Can you work these out from the model? Positions are in its coordinate system, mm. A direction names the side the tool comes from. Give positions to 0.01 mm unless a question says otherwise; leave off trailing zeros. Answer as a JSON object with one key per item and string values.
Autodesk Inventor part; units mm, degrees
ref_plane "YZ Plane" through (0, 0, 0) normal (1, 0, 0) x (0, 1, 0)
ref_plane "XZ Plane" through (0, 0, 0) normal (0, 1, 0) x (-1, 0, 0)
ref_plane "XY Plane" through (0, 0, 0) normal (0, 0, 1) x (1, 0, 0)
sketch "Szkic1" plane through (0, 0, 0) normal (0, 1, 0) x (-1, 0, 0)
  line L0 (35.259, 49.5664) -> (-29.741, 49.5664)
  line L1 (-29.741, 49.5664) -> (-29.741, 19.5664)
  line L2 (-29.741, 19.5664) -> (35.259, 19.5664)
  line L3 (35.259, 19.5664) -> (35.259, 49.5664)
  point P0 (0, 0)
  dimension "d0" = 65
  dimension "d1" = 30
extrude "Wyciągnięcie proste1" add sketch "Szkic1" along normal blind 1.6
fillet "Zaokrąglenie1" radius 2 4 edges at (-35.259, 0.8, 19.5664) (-35.259, 0.8, 49.5664) (29.741, 0.8, 49.5664) (29.741, 0.8, 19.5664)
sketch "Szkic2" plane through (0, 1.6, 0) normal (0, 1, 0) x (1, 0, 0)
  arc A0 (29.741, -21.5664) -> (27.741, -19.5664) centre (27.741, -21.5664) ccw
  line L0 (27.741, -19.5664) -> (-33.259, -19.5664)
  arc A1 (-33.259, -19.5664) -> (-35.259, -21.5664) centre (-33.259, -21.5664) ccw
  line L1 (-35.259, -21.5664) -> (-35.259, -47.5664)
  arc A2 (-35.259, -47.5664) -> (-33.259, -49.5664) centre (-33.259, -47.5664) ccw
  line L2 (-33.259, -49.5664) -> (27.741, -49.5664)
  arc A3 (27.741, -49.5664) -> (29.741, -47.5664) centre (27.741, -47.5664) ccw
  line L3 (29.741, -47.5664) -> (29.741, -21.5664)
  line L4 (-33.259, -20.0664) -> (27.741, -20.0664)
  arc A4 (29.241, -21.5664) -> (27.741, -20.0664) centre (27.741, -21.5664) ccw
  line L5 (29.241, -21.5664) -> (29.241, -47.5664)
  arc A5 (27.741, -49.0664) -> (29.241, -47.5664) centre (27.741, -47.5664) ccw
  line L6 (27.741, -49.0664) -> (-33.259, -49.0664)
  arc A6 (-34.759, -47.5664) -> (-33.259, -49.0664) centre (-33.259, -47.5664) ccw
  line L7 (-34.759, -47.5664) -> (-34.759, -21.5664)
  arc A7 (-33.259, -20.0664) -> (-34.759, -21.5664) centre (-33.259, -21.5664) ccw
  point P0 (0, 0)
  dimension "d5" = 0.5
extrude "Wyciągnięcie proste2" cut sketch "Szkic2" against normal through all
sketch "Szkic3" plane through (0, 1.6, 0) normal (0, 1, 0) x (1, 0, 0)
  line L0 (-19.799, -32.0164) -> (-20.439, -32.0164)
  line L1 (-20.439, -32.0164) -> (-20.439, -31.3764)
  line L2 (-19.799, -31.3764) -> (-19.799, -32.0164)
  line L3 (-20.439, -31.3764) -> (-19.799, -31.3764)
  line L4 (-19.799, -29.4764) -> (-20.439, -29.4764)
  line L5 (-19.799, -28.8364) -> (-19.799, -29.4764)
  line L6 (-20.439, -29.4764) -> (-20.439, -28.8364)
  line L7 (-20.439, -28.8364) -> (-19.799, -28.8364)
  line L8 (-19.799, -26.9364) -> (-20.439, -26.9364)
  line L9 (-19.799, -26.2964) -> (-19.799, -26.9364)
  line L10 (-20.439, -26.9364) -> (-20.439, -26.2964)
  line L11 (-20.439, -26.2964) -> (-19.799, -26.2964)
  line L12 (-20.439, -24.3964) -> (-20.439, -23.7564)
  line L13 (-19.799, -24.3964) -> (-20.439, -24.3964)
  line L14 (-20.439, -23.7564) -> (-19.799, -23.7564)
  line L15 (-19.799, -23.7564) -> (-19.799, -24.3964)
  line L16 (-17.469, -25.4431) -> (-16.829, -25.4431)
  line L17 (-17.469, -26.0831) -> (-17.469, -25.4431)
  line L18 (-16.829, -26.0831) -> (-17.469, -26.0831)
  line L19 (-16.829, -25.4431) -> (-16.829, -26.0831)
  line L20 (-14.929, -26.0831) -> (-14.929, -25.4431)
  line L21 (-14.289, -26.0831) -> (-14.929, -26.0831)
  line L22 (-14.929, -25.4431) -> (-14.289, -25.4431)
  line L23 (-14.289, -25.4431) -> (-14.289, -26.0831)
  line L24 (-12.389, -26.0831) -> (-12.389, -25.4431)
  line L25 (-11.749, -26.0831) -> (-12.389, -26.0831)
  line L26 (-12.389, -25.4431) -> (-11.749, -25.4431)
  line L27 (-11.749, -25.4431) -> (-11.749, -26.0831)
  line L28 (-9.849, -26.0831) -> (-9.849, -25.4431)
  line L29 (-9.209, -25.4431) -> (-9.209, -26.0831)
  line L30 (-9.849, -25.4431) -> (-9.209, -25.4431)
  line L31 (-9.209, -26.0831) -> (-9.849, -26.0831)
  line L32 (-2.759, -11.5664) -> (-2.759, -67.5664)
  line L33 (-34.259, -33.2664) -> (-32.659, -33.2664)
  line L34 (-34.259, -33.2664) -> (-34.259, -22.5664)
  line L35 (-34.259, -22.5664) -> (-32.659, -22.5664)
  line L36 (-32.659, -22.5664) -> (-32.659, -33.2664)
  line L37 (-34.259, -33.2664) -> (-32.659, -33.2664)
  line L38 (-7.959, -39.9031) -> (-18.659, -39.9031)
  line L39 (-18.659, -39.9031) -> (-18.659, -38.3031)
  line L40 (-18.659, -38.3031) -> (-7.959, -38.3031)
  line L41 (-7.959, -39.9031) -> (-7.959, -38.3031)
  line L42 (2.441, -39.9031) -> (13.141, -39.9031)
  line L43 (2.441, -39.9031) -> (2.441, -38.3031)
  line L44 (13.141, -38.3031) -> (2.441, -38.3031)
  line L45 (13.141, -39.9031) -> (13.141, -38.3031)
  line L46 (28.741, -33.2664) -> (28.741, -22.5664)
  line L47 (28.741, -33.2664) -> (27.141, -33.2664)
  line L48 (27.141, -22.5664) -> (27.141, -33.2664)
  line L49 (28.741, -22.5664) -> (27.141, -22.5664)
  line L50 (14.281, -32.0164) -> (14.921, -32.0164)
  line L51 (14.921, -32.0164) -> (14.921, -31.3764)
  line L52 (14.281, -31.3764) -> (14.281, -32.0164)
  line L53 (14.921, -31.3764) -> (14.281, -31.3764)
  line L54 (14.281, -29.4764) -> (14.921, -29.4764)
  line L55 (14.281, -28.8364) -> (14.281, -29.4764)
  line L56 (14.921, -29.4764) -> (14.921, -28.8364)
  line L57 (14.921, -28.8364) -> (14.281, -28.8364)
  line L58 (14.281, -26.9364) -> (14.921, -26.9364)
  line L59 (14.281, -26.2964) -> (14.281, -26.9364)
  line L60 (14.921, -26.9364) -> (14.921, -26.2964)
  line L61 (14.921, -26.2964) -> (14.281, -26.2964)
  line L62 (14.921, -24.3964) -> (14.921, -23.7564)
  line L63 (14.281, -24.3964) -> (14.921, -24.3964)
  line L64 (14.921, -23.7564) -> (14.281, -23.7564)
  line L65 (14.281, -23.7564) -> (14.281, -24.3964)
  line L66 (11.951, -25.4431) -> (11.311, -25.4431)
  line L67 (11.951, -26.0831) -> (11.951, -25.4431)
  line L68 (11.311, -26.0831) -> (11.951, -26.0831)
  line L69 (11.311, -25.4431) -> (11.311, -26.0831)
  line L70 (9.411, -26.0831) -> (9.411, -25.4431)
  line L71 (8.771, -26.0831) -> (9.411, -26.0831)
  line L72 (9.411, -25.4431) -> (8.771, -25.4431)
  line L73 (8.771, -25.4431) -> (8.771, -26.0831)
  line L74 (6.871, -26.0831) -> (6.871, -25.4431)
  line L75 (6.231, -26.0831) -> (6.871, -26.0831)
  line L76 (6.871, -25.4431) -> (6.231, -25.4431)
  line L77 (6.231, -25.4431) -> (6.231, -26.0831)
  line L78 (4.331, -26.0831) -> (4.331, -25.4431)
  line L79 (3.691, -25.4431) -> (3.691, -26.0831)
  line L80 (4.331, -25.4431) -> (3.691, -25.4431)
  line L81 (3.691, -26.0831) -> (4.331, -26.0831)
  arc A0 (-33.259, -20.0664) -> (-34.759, -21.5664) centre (-33.259, -21.5664) ccw
  line L82 (-34.759, -21.5664) -> (-34.759, -47.5664)
  arc A1 (-34.759, -47.5664) -> (-33.259, -49.0664) centre (-33.259, -47.5664) ccw
  line L83 (-33.259, -49.0664) -> (27.741, -49.0664)
  arc A2 (27.741, -49.0664) -> (29.241, -47.5664) centre (27.741, -47.5664) ccw
  line L84 (29.241, -47.5664) -> (29.241, -21.5664)
  arc A3 (29.241, -21.5664) -> (27.741, -20.0664) centre (27.741, -21.5664) ccw
  line L85 (27.741, -20.0664) -> (-33.259, -20.0664)
  line L86 (-32.359, -33.2664) -> (-32.359, -22.2664)
  line L87 (-32.359, -22.2664) -> (-34.559, -22.2664)
  line L88 (-34.559, -22.2664) -> (-34.559, -33.2664)
  line L89 (-34.259, -33.5664) -> (-32.659, -33.5664)
  line L90 (-34.559, -22.2664) -> (-32.359, -22.2664)
  line L91 (-32.359, -22.2664) -> (-32.359, -33.5664)
  line L92 (-32.359, -33.5664) -> (-34.559, -33.5664)
  line L93 (-34.559, -33.5664) -> (-34.559, -22.2664)
  line L94 (-18.959, -40.2031) -> (-7.659, -40.2031)
  line L95 (-7.659, -40.2031) -> (-7.659, -38.0031)
  line L96 (-7.659, -38.0031) -> (-18.959, -38.0031)
  line L97 (-18.959, -38.0031) -> (-18.959, -40.2031)
  line L98 (13.441, -40.2031) -> (2.141, -40.2031)
  line L99 (2.141, -40.2031) -> (2.141, -38.0031)
  line L100 (2.141, -38.0031) -> (13.441, -38.0031)
  line L101 (13.441, -38.0031) -> (13.441, -40.2031)
  line L102 (26.841, -33.5664) -> (29.041, -33.5664)
  line L103 (29.041, -33.5664) -> (29.041, -22.2664)
  line L104 (29.041, -22.2664) -> (26.841, -22.2664)
  line L105 (26.841, -22.2664) -> (26.841, -33.5664)
  point P0 (0, 0)
  dimension "d8" = 0.3
  dimension "d9" = 0.3
  dimension "d10" = 0.3
  dimension "d11" = 0.3
  dimension "d12" = 0.3
extrude "Wyciągnięcie proste3" cut sketch "Szkic3" against normal through all contours L0 L1 L3 L2 | L4 L6 L7 L5 | L8 L10 L11 L9 | L12 L14 L15 L13 | L16 L19 L18 L17 | L20 L22 L23 L21 | L24 L26 L27 L25 | L28 L30 L29 L31 | L34 L35 L36 L33 | L38 L39 L40 L41 | L43 L44 L45 L42 | L47 L48 L49 L46 | L52 L53 L51 L50 | L55 L57 L56 L54 | L59 L61 L60 L58 | L63 L65 L64 L62 | L67 L68 L69 L66 | L71 L73 L72 L70 | L75 L77 L76 L74 | L81 L79 L80 L78 | L91 L92 L89 L93 L88 L87 L86 | L97 L96 L95 L94 | L98 L99 L100 L101 | L105 L104 L103 L102
properties part number "MS_PCB"
1) If we mould it in two halves opening along X, with no side actions, what happens to faces 1 (the flat face through (-2, 0, 35)), 2 (the cylindrical face through (-34.331, 0.811, 48.615)), 3 (the flat face through (-13, 1, 40.203)), 4 (the flat face through (-18.959, 1, 39))? For each: +X half, -X half, draft (parallel to the pull), parting line (faces both ways), or undercut.
Answer list:
{"face 1": "draft", "face 2": "-X half", "face 3": "undercut", "face 4": "undercut"}
2) Please list where these lines run through material, in increasing order: line 1 along Z through (x, y) = (11.5, 0.15); line 2 along X through (y, z) = (0.6, 33.5); line 3 along X through (y, z) = (0.9, 39.5). Write a range as from..to.
Answer list:
{"line 1": "20.07..25.44, 26.08..38, 40.2..49.07", "line 2": "-34.76..-34.56, -32.36..26.84, 29.04..29.24", "line 3": "-34.76..-18.96, -7.66..2.14, 13.44..29.24"}
3) Suppose I cut it at A-A, the plane y = 1. Give the number of separate pieces and of enclosed holes in the cut face, and give its area (3 significant figures).
Answer list:
{"separate pieces": "1", "enclosed holes": "20", "area": "1,750 mm^2"}
4) For faces 5 (the flat face through (-34.759, 1, 35)), 6 (the flat face through (2.141, 1, 39)), which set-ups out of +Z, -Z, +X, -X, +Y, -Y let a thin tool reach every point of the face, with its end or its side?
Answer list:
{"face 5": "+Z, -Z, -X, +Y, -Y", "face 6": "+Y, -Y"}
